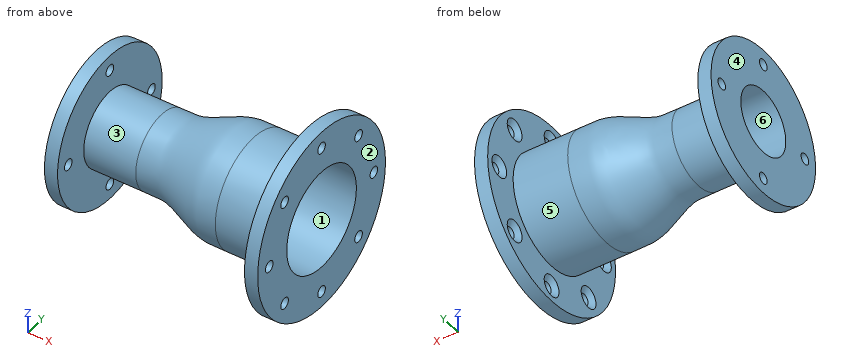
```python
from build123d import *

# Parameters (mm, degrees)
F_5_8_CLEARANCE_HOLE1_D                             = 16.66748
F_5_8_CLEARANCE_HOLE1_DEPTH                         = 20
CSK_FOR_5_8_FLAT_HEAD_MACHINE_SCREW_100_D           = 16.66748
CSK_FOR_5_8_FLAT_HEAD_MACHINE_SCREW_100_DEPTH       = 20
CSK_FOR_5_8_FLAT_HEAD_MACHINE_SCREW_100_CSINK_D     = 32.3088
CSK_FOR_5_8_FLAT_HEAD_MACHINE_SCREW_100_CSINK_ANGLE = 100


with BuildPart() as part:
    # Sketch2 → Revolve1 (revolve)
    with BuildSketch(Plane.XY):
        with BuildLine():
            Line((341.7, 76.137499212), (341.7, 139.7))
            Line((341.7, 139.7), (321.7, 139.7))
            Line((321.7, 139.7), (321.7, 84.137499212))
            Line((321.7, 84.137499212), (238.7, 84.137499212))
            add(Edge.make_bspline(
                [(238.7, 84.137499212), (238.355924075, 84.137499212), (237.667772223, 84.137499211), (236.43892963, 84.137499212), (234.866011112, 84.137499209), (233.096477778, 84.137499221), (231.179483334, 84.137499181), (229.409949997, 84.137499346), (227.492955565, 84.137498785), (225.723422181, 84.137501116), (223.806427909, 84.137493202), (222.03689386, 84.137526067), (220.119901847, 84.137414453), (218.350358415, 84.137877999), (216.436180482, 84.136306025), (214.671251811, 84.142808495), (212.761120781, 84.086749305), (210.997970421, 83.981894478), (209.088061418, 83.811610968), (207.325068085, 83.603702947), (205.415339805, 83.325577691), (203.652528826, 83.021476856), (201.742980231, 82.643054651), (199.980349522, 82.250081454), (198.070973132, 81.779589057), (196.308510241, 81.305636666), (194.399291637, 80.751921317), (192.636978054, 80.205434277), (190.727898375, 79.577923288), (188.965712472, 78.967858654), (187.056750607, 78.276511422), (185.294669761, 77.61229035), (183.385803915, 76.867540678), (181.623805854, 76.15899109), (179.715014471, 75.371680114), (177.95307795, 74.628970979), (176.044340155, 73.810271455), (174.28244512, 73.043839656), (172.373740784, 72.205172954), (170.611868192, 71.425644088), (168.701772289, 70.577967809), (166.937395899, 69.794959659), (165.024786727, 68.949453647), (163.259291454, 68.174390413), (161.346657228, 67.343861664), (159.58112861, 66.587981326), (157.668449277, 65.784003027), (155.902867536, 65.057899506), (153.990122343, 64.291832507), (152.22446654, 63.60586364), (150.311633974, 62.888769921), (148.545882008, 62.252980739), (146.632940071, 61.595543531), (144.867069113, 61.019596499), (142.95399603, 60.432048638), (141.187983586, 59.925161995), (139.274759098, 59.417223546), (137.508584813, 58.988118492), (135.595192141, 58.568944237), (133.828840435, 58.225800875), (131.915268777, 57.903938632), (130.148732425, 57.654357312), (128.234978669, 57.437727635), (126.468267149, 57.288649922), (124.789582716, 57.197477456), (123.443760708, 57.156958736), (122.420535806, 57.149027418), (121.677966993, 57.150148752), (120.601758891, 57.149831794), (119.202172332, 57.150049881), (117.285177742, 57.149983489), (115.515644452, 57.150003038), (113.598649997, 57.149998331), (111.829116667, 57.149999717), (109.912122221, 57.149999383), (108.142588888, 57.149999482), (106.225594444, 57.149999458), (104.45606111, 57.149999465), (102.539066666, 57.149999463), (101.039878703, 57.149999464), (99.81103611, 57.149999464), (99.27034537, 57.149999464), (98.999999999, 57.149999464)],
                knots=[0, 0, 0, 0, 0.007154165, 0.014308329, 0.025550588, 0.039858917, 0.051101176, 0.065409505, 0.076651764, 0.090960094, 0.102202352, 0.116510682, 0.12775294, 0.14206127, 0.153303528, 0.167554008, 0.178755429, 0.193030915, 0.204271905, 0.218620642, 0.229935227, 0.24439542, 0.255809505, 0.270408809, 0.281939941, 0.296695409, 0.308352907, 0.323271342, 0.335056718, 0.350135378, 0.362042998, 0.377270556, 0.389288475, 0.404646168, 0.416757099, 0.432220021, 0.44440238, 0.459940864, 0.472169892, 0.487750951, 0.499999862, 0.51562065, 0.52788688, 0.543480107, 0.55571106, 0.571242545, 0.583412274, 0.598850533, 0.610935794, 0.626253518, 0.638234915, 0.653410393, 0.66527347, 0.680291945, 0.692028204, 0.706883096, 0.718490902, 0.733184872, 0.744670204, 0.75921598, 0.770592966, 0.785013865, 0.796305044, 0.810635098, 0.821871343, 0.831256632, 0.838627865, 0.843146285, 0.846696472, 0.861004801, 0.87224706, 0.886555389, 0.897797648, 0.912105977, 0.923348236, 0.937656565, 0.948898824, 0.963207153, 0.974449412, 0.988757741, 0.994378871, 1, 1, 1, 1], degree=3, weights=[0.576132148, 0.576132148, 0.576132148, 0.576132148, 0.576132148, 0.576132148, 0.576132148, 0.576132148, 0.576132148, 0.576132148, 0.576132148, 0.576132148, 0.576132148, 0.576132148, 0.576132148, 0.576132148, 0.576132148, 0.576132148, 0.576132148, 0.576132148, 0.576132148, 0.576132148, 0.576132148, 0.576132148, 0.576132148, 0.576132148, 0.576132148, 0.576132148, 0.576132148, 0.576132148, 0.576132148, 0.576132148, 0.576132148, 0.576132148, 0.576132148, 0.576132148, 0.576132148, 0.576132148, 0.576132148, 0.576132148, 0.576132148, 0.576132148, 0.576132148, 0.576132148, 0.576132148, 0.576132148, 0.576132148, 0.576132148, 0.576132148, 0.576132148, 0.576132148, 0.576132148, 0.576132148, 0.576132148, 0.576132148, 0.576132148, 0.576132148, 0.576132148, 0.576132148, 0.576132148, 0.576132148, 0.576132148, 0.576132148, 0.576132148, 0.576132148, 0.576132148, 0.576132148, 0.576132148, 0.576132148, 0.576132148, 0.576132148, 0.576132148, 0.576132148, 0.576132148, 0.576132148, 0.576132148, 0.576132148, 0.576132148, 0.576132148, 0.576132148, 0.576132148, 0.576132148, 0.576132148]))
            Line((98.999999999, 57.149999464), (20, 57.149999464))
            Line((20, 57.149999464), (20, 114.3))
            Line((20, 114.3), (0, 114.3))
            Line((0, 114.3), (0, 49.149999464))
            Line((0, 49.149999464), (98.999999999, 49.149999464))
            add(Edge.make_bspline(
                [(238.700000001, 76.137499212), (235.69409428, 76.137499211), (231.185175342, 76.137529978), (225.92498116, 76.137458281), (222.918904328, 76.137568327), (220.664664612, 76.137283149), (218.784669959, 76.138023248), (217.290602157, 76.13677783), (216.128457097, 76.1382361), (215.066881493, 76.138852647), (213.792519107, 76.118938664), (211.496695076, 76.015652057), (208.229301379, 75.6893674), (204.270612611, 75.027164667), (200.298712296, 74.120693109), (194.985358164, 72.623109637), (188.321466773, 70.283294689), (180.275439823, 66.96143105), (172.126179657, 63.34551056), (163.790302615, 59.64532736), (155.164556548, 56.079333574), (147.64132386, 53.429737774), (141.378908996, 51.662061148), (136.556364248, 50.559794229), (131.615917341, 49.730227773), (127.403841781, 49.309288048), (124.437765649, 49.174559905), (122.930150126, 49.151400947), (122.100741829, 49.149426118), (121.356980871, 49.150399773), (120.417271001, 49.149754665), (118.913072261, 49.150117503), (117.035873074, 49.149952223), (114.780889972, 49.150013449), (111.775161973, 49.149990987), (106.514717734, 49.150005821), (102.005905795, 49.149999464), (98.999999999, 49.149999464)],
                knots=[0, 0, 0, 0, 0.0625, 0.09375, 0.109375, 0.125, 0.140625, 0.1484375, 0.15625, 0.1640625, 0.171875, 0.1875, 0.21875, 0.25, 0.28125, 0.3125, 0.375, 0.4375, 0.5, 0.5625, 0.625, 0.6875, 0.71875, 0.75, 0.78125, 0.8125, 0.828125, 0.8359375, 0.83984375, 0.84375, 0.8515625, 0.859375, 0.875, 0.890625, 0.90625, 0.9375, 1, 1, 1, 1], degree=3))
            Line((238.700000001, 76.137499212), (341.7, 76.137499212))
        make_face()
    revolve(axis=Axis((341.7, 0, 0), (-1, 0, 0)))

    # 5/8 Clearance Hole1
    with Locations(Plane(origin=(0, -86.94526051, 61.229912904), x_dir=(0, 0, 1), z_dir=(-1, 0, 0))):
        with Locations((-61.229912904, 177.798020209), (29.681467244, 86.94526051), (-61.229912904, -3.966119638), (-152.141293051, 86.94526051)):
            Hole(F_5_8_CLEARANCE_HOLE1_D / 2, depth=F_5_8_CLEARANCE_HOLE1_DEPTH)

    # CSK for 5_8 Flat Head Machine Screw _100
    with Locations(Plane(origin=(321.7, -86.94526051, 61.229912904), x_dir=(0, 0, 1), z_dir=(-1, 0, 0))):
        with Locations((-61.229912904, 201.24526051), (-176.596487394, 86.94526051), (-142.052217993, 167.767565599), (19.592392186, 167.767565599), (53.070087096, 86.94526051), (19.592392186, 6.12295542), (-61.229912904, -27.406492985), (-142.052217993, 6.12295542)):
            CounterSinkHole(CSK_FOR_5_8_FLAT_HEAD_MACHINE_SCREW_100_D / 2, CSK_FOR_5_8_FLAT_HEAD_MACHINE_SCREW_100_CSINK_D / 2, depth=CSK_FOR_5_8_FLAT_HEAD_MACHINE_SCREW_100_DEPTH, counter_sink_angle=CSK_FOR_5_8_FLAT_HEAD_MACHINE_SCREW_100_CSINK_ANGLE)


solid = part.part
```
The listing builds one solid part. Answer for the finished solid, in the listing's coordinates (mm). Face numbers are marked on the shaded views. A direction names the side the tool comes from. Round coordinates to 2 decimals unless told otherwise and drop trailing zeros.
Q1. Given pin 1 Ø10 at (y, z) = (90.85, 0) entering from -X; pin 2 Ø8 at (y, z) = (-34, 50) entering from +X; pin 3 Ø13.5 at (y, z) = (114.3, 0) entering from +X; pin 4 Ø3 at (y, z) = (-16, 43.5) entering from -X, each flat-ended and moving along its own axis, determine where each tip first touches the part or whether it passes through.
Q2. Find the intervals of material crossed by line 1 (Y direction, x = 333, z = 0); line 2 (X direction, y = 84, z = 15.5); line 3 (Z direction, x = 336, y = 0), in increasing order.
Q3. Which of the six approach directions +Z, -Z, +X, -X, +Y, -Y give full straight-line access (tool end or side, diameter ignored) to the marked faces 5 and 6?
Q4. For a pull along X with two mould halves and no side action, classify the marked faces 1, 2, 3 and 4 as released by +X, released by -X, zero draft, split by the parting line, or undercut.
Q5. Section A-A, the plane y = 0 is taken. Count the separate pieces of the cut face and the enclosed holes in it, then the cut area to 3 significant figures.
Completed:
1. pin 1: stops at x = 321.7
1. pin 2: stops at x = 174.65
1. pin 3: stops at x = 20
1. pin 4: passes through
2. line 1: y = -139.7 to -122.69, -106.02 to -76.14, 76.14 to 105.97, 122.63 to 139.7
2. line 2: x = 0 to 20, 321.7 to 341.7
2. line 3: z = -139.7 to -123.7, -107.03 to -76.14, 76.14 to 105.97, 122.63 to 139.7
3. face 5: none
3. face 6: +X, -X
4. face 1: zero draft
4. face 2: released by +X
4. face 3: undercut
4. face 4: released by -X
5. separate pieces: 6
5. enclosed holes: 0
5. area: 8,610 mm2
